For this review, take the finished solid that the model builds, in its own axes (mm). A direction names the side the tool comes from. Round coordinates to 2 decimals unless told otherwise and drop trailing zeros. Write each loop counter-clockwise with the first axis right and the second up, starting at its lowest first coordinate (ties: lowest second). Pieces come first, ordered by that corner, then holes. Notation, with made-up numbers: M -33,88.5 L 9,88.5 A28 cw 9,126.5 Z; hole C -40,52.5 d11. An arc over 180 degrees is marked long. Use one line per item in the form item = value. Start each with the question number.
Item 1: Draft analysis for pull direction Y (two halves, no side actions). For faces 1 (the flat face through (-9.583, 0.787, 15.957)), 2 (the flat face through (0, -9.25, 111)), 3 (the flat face through (0, 10, 100)), 4 (the flat face through (-9.25, 0, 100)), state which applies: released by +Y, released by -Y, zero draft, split by the parting line, or undercut.
Item 2: Add section B-B (z = 90). State the section outline as (x, y) points.
Item 3: For faces 5 (the flat face through (0, 9.25, 100)), 6 (the flat face through (-10, 0, 100)), list the 3-axis set-ups (+Z, -Z, +X, -X, +Y, -Y) from which the entire face can be reached by the end or side of a thin tool; tool diameter is ignored.
Item 4: Add section C-C (y = -5). State the section outline as (x, z) points.
Item 5: For line 1 (Y direction, x = -0.5, z = 124); line 2 (Y direction, x = -6, z = 18), list the stretches that pass through material, from the lowest coordinate up. Write a range as [from, to].
Item 6: Add section A-A (x = -4.5). State the section outline as (y, z) points.
Item 7: For P1, Ø3, axis at x = 0, y = 8, coming from the -Z side; P2, Ø8, axis at x = -1.5, y = -7, coming from the +Z side, all flat-tipped, find the tip position at first contact; note any pin that passes through.
Autodesk Inventor part; units mm, degrees
ref_plane "YZ Plane" through (0, 0, 0) normal (1, 0, 0) x (0, 1, 0)
ref_plane "XZ Plane" through (0, 0, 0) normal (0, 1, 0) x (-1, 0, 0)
ref_plane "XY Plane" through (0, 0, 0) normal (0, 0, 1) x (1, 0, 0)
sketch "Эскиз1" plane through (0, 0, 0) normal (0, 0, 1) x (1, 0, 0)
  line L0 (10, -10) -> (-10, -10)
  line L1 (-10, -10) -> (-10, 10)
  line L2 (-10, 10) -> (10, 10)
  line L3 (10, 10) -> (10, -10)
  line L4 (10, -10) -> (-10, 10) construction
  line L5 (-10, -10) -> (10, 10) construction
  line L6 (9.25, -9.25) -> (-9.25, -9.25)
  line L7 (-9.25, -9.25) -> (-9.25, 9.25)
  line L8 (-9.25, 9.25) -> (9.25, 9.25)
  line L9 (9.25, 9.25) -> (9.25, -9.25)
  line L10 (9.25, -9.25) -> (-9.25, 9.25) construction
  line L11 (-9.25, -9.25) -> (9.25, 9.25) construction
  point P0 (0, 0)
  dimension "d0" = 20
  dimension "d1" = 20
  dimension "d2" = 18.5
  dimension "d3" = 18.5
extrude "Выдавливание1" add sketch "Эскиз1" along normal blind 202.0726
sketch "Эскиз2" plane through (10, -10, 0) normal (1, 0, 0) x (0, 0, -1)
  line L0 (0, 0) -> (0, 20)
  line L1 (0, 20) -> (-34.641, 0)
  line L2 (0, 0) -> (-202.0726, 0)
  line L3 (0, 20) -> (40, 20) construction
  line L4 (-34.641, 0) -> (0, 0)
  line L5 (0, 0) -> (0, 20)
  point P0 (0, 10)
  dimension "d6" = 150
extrude "Выдавливание2" cut sketch "Эскиз2" against normal blind 178.9786
sketch "Эскиз3" plane through (10, -10, 202.0726) normal (1, 0, 0) x (0, 0, -1)
  line L0 (0, 20) -> (11.547, 0)
  line L1 (167.4316, 0) -> (0, 0)
  line L2 (0, 20) -> (23.094, 20) construction
  line L3 (11.547, 0) -> (0, 0)
  line L4 (0, 0) -> (0, 20)
  line L5 (0, 0) -> (0, 20)
  point P0 (202.0726, 10)
  dimension "d9" = 60
extrude "Выдавливание3" cut sketch "Эскиз3" against normal blind 202.0726
Calculated:
q1.face_1 = released by -Y
q1.face_2 = undercut
q1.face_3 = released by +Y
q1.face_4 = undercut
q2.outline = M -10,-10 L 10,-10 L 10,10 L -10,10 Z; hole M -9.25,-9.25 L 9.25,-9.25 L 9.25,9.25 L -9.25,9.25 Z
q3.face_5 = +Z, -Z
q3.face_6 = +Z, -Z, -X, +Y, -Y
q4.outline = M -10,25.98 L -9.25,25.98 L -9.25,193.41 L -10,193.41 Z; M 9.25,25.98 L 10,25.98 L 10,193.41 L 9.25,193.41 Z
q5.line_1 = [-10, -9.25], [9.25, 10]
q5.line_2 = [9.25, 10]
q6.outline = M -10,34.64 L -9.25,33.34 L -9.25,190.96 L -10,190.53 Z; M 9.25,1.3 L 10,0 L 10,202.07 L 9.25,201.64 Z
q7.P1 = 0.87
q7.P2 = 190.96
